Source: CAD feature listing. Evaluate the final solid. Frame: model axes, mm. A direction names the side the tool comes from. Round coordinates to 2 decimals unless told otherwise and drop trailing zeros. Loops run counter-clockwise (first coordinate to the right, second up) from the corner with the lowest first, then second, coordinate; pieces in that order, holes last. Notation, with made-up numbers: (-16, 48) -> (-1, 48) arc R28 ccw to (-1, 75) -> close; hole circle Ø9 at (81, -35.75). An arc over 180 degrees is marked (long way). Put each result on its own line as item: value. Start each with the question number.
1. Cut plane D-D (y = 7.5). Return the cut outline in (x, z), then the cut area to 3 significant figures.
2. Cut plane C-C (z = -1). State how many separate pieces and enclosed holes the cut face has, then the cut area to 3 significant figures.
3. Contact query for flat-ended pins moving along their axis: pin 1 (4 mm diameter, centred on y = -13.5, z = -3, fed in from +X); pin 2 (2.5 mm diameter, centred on x = -25, z = -3.5, fed in from -Y); pin 3 (4 mm diameter, centred on x = -26, z = -3, fed in from +Y). Output: stop coordinate, or through.
4. Cut plane B-B (x = -9). Return the cut outline in (y, z).
5. Draft query along Y for faces 1 (the cylindrical face through (21.37, 11.23, 8.55)), 2 (the cylindrical face through (-24.503, -13.631, 8.549)), 3 (the flat face through (0, -20, 4)), 4 (the cylindrical face through (-12.41, -16.07, 7.75)). Return one class per face: pulls with the +Y half, pulls with the -Y half, needs draft (parallel to the pull), parting line crosses it, or undercut.
6. Set-up query: faces 5 (the flat face through (10, 14, 3)), 6 (the flat face through (12.3, 4, 6.6)), 7 (the cylindrical face through (-7.9, -17.97, -1.09)). Return all of +Z, -Z, +X, -X, +Y, -Y with unobstructed straight access to the full face (end or side cutting, diameter ignored); none if empty.
7. Material intervals for L1, parallel to X at y = 13, z = -2; L2, parallel to X at y = -13, z = 0.5; L3, parallel to Y at x = -22.5, z = 8, sorted ascending.
8. Cut plane A-A (y = -1). Return the cut outline in (x, z), then the cut area to 3 significant figures.
```python
from build123d import *
from build123d.topology import SkipClean

# Parameters (mm, degrees)
ESQUISSE1_W                  = 55
ESQUISSE1_H                  = 45
BOSS_EXTRU_1_DEPTH           = 12
ESQUISSE2_R                  = 4.25
ENL_V_MAT_EXTRU_1_DEPTH      = 55.085580333
ENL_V_MAT_EXTRU_2_DEPTH      = 12.25
ENL_V_MAT_EXTRU_2_DEPTH_BACK = 12.25
ESQUISSE3_R                  = 7.75
ESQUISSE9_W                  = 61.062756781
ESQUISSE9_H                  = 12.22812859
ESQUISSE9_W_2                = 59.427147224
ESQUISSE9_H_2                = 8.100161614
ENL_V_MAT_EXTRU_7_DEPTH      = 31
SKETCH1_W                    = 55
SKETCH1_H                    = 36
BOSS_EXTRUDE1_DEPTH          = 5
SKETCH2_R                    = 2.1
CUT_EXTRUDE1_DEPTH           = 38.003378224
SKETCH3_R                    = 4
CUT_EXTRUDE2_DEPTH           = 10
CUT_EXTRUDE3_DEPTH           = 5
SKETCH5_R                    = 2.1
CUT_EXTRUDE4_DEPTH           = 47.864165415
BOSS_EXTRUDE4_START          = 2
SKETCH7_R                    = 2.1
BOSS_EXTRUDE4_DEPTH          = 2
SKETCH8_R                    = 2.1
BOSS_EXTRUDE5_DEPTH          = 2
SKETCH9_W                    = 7
SKETCH9_H                    = 3.2
CUT_EXTRUDE6_DEPTH           = 8
SKETCH10_W                   = 4.25
SKETCH10_H                   = 4
SKETCH10_H_2                 = 2
SKETCH10_H_3                 = 10
SKETCH10_W_2                 = 0.75


with BuildPart() as part:
    # Esquisse1 → Boss.-Extru.1 (new body)
    with BuildSketch(Plane.XY):
        Rectangle(ESQUISSE1_W, ESQUISSE1_H)
    extrude(amount=BOSS_EXTRU_1_DEPTH)

    # Esquisse2 → Enl_v. mat.-Extru.1 (cut, through all)
    with BuildSketch(Plane(origin=(0, 22.5, 0), x_dir=(1, 0, 0), z_dir=(0, 1, 0))):
        with Locations((-12.5, -12)):
            Circle(ESQUISSE2_R)
        with Locations((12.5, -12)):
            Circle(ESQUISSE2_R)
    extrude(amount=-ENL_V_MAT_EXTRU_1_DEPTH, mode=Mode.SUBTRACT)

    # Esquisse3 → Enl_v. mat.-Extru.2 (cut, two sides: drawn at the far end of the back side and taken through both)
    with BuildSketch(Plane(origin=(0, 0, 0), x_dir=(1, 0, 0), z_dir=(0, 1, 0)).offset(-ENL_V_MAT_EXTRU_2_DEPTH_BACK)):
        with Locations((-12.5, -12)):
            Circle(ESQUISSE3_R)
    extrude(amount=ENL_V_MAT_EXTRU_2_DEPTH + ENL_V_MAT_EXTRU_2_DEPTH_BACK, mode=Mode.SUBTRACT)

    # Esquisse9 → Enl_v. mat.-Extru.7 (cut)
    with BuildSketch(Plane.XY.offset(12)):
        with Locations((-0.389430846, -24.114064295)):
            Rectangle(ESQUISSE9_W, ESQUISSE9_H)
        with Locations((1.674552641, 22.050080807)):
            Rectangle(ESQUISSE9_W_2, ESQUISSE9_H_2)
    extrude(amount=-ENL_V_MAT_EXTRU_7_DEPTH, mode=Mode.SUBTRACT)

    # Sketch1 → Boss-Extrude1 (add)
    with BuildSketch(Plane(origin=(0, 0, 0), x_dir=(-1, 0, 0), z_dir=(0, 0, -1))):
        Rectangle(SKETCH1_W, SKETCH1_H)
    extrude(amount=BOSS_EXTRUDE1_DEPTH)

    # Sketch2 → Cut-Extrude1 (cut, through all)
    with BuildSketch(Plane.XY.offset(12)):
        with Locations((-22.5, 13)):
            Circle(SKETCH2_R)
        with Locations(Location((22.5, 13, 0), (0, 0, 180))):
            Circle(SKETCH2_R)
        with Locations((22.5, -13)):
            Circle(SKETCH2_R)
        with Locations(Location((-22.5, -13, 0), (0, 0, 180))):
            Circle(SKETCH2_R)
    extrude(amount=-CUT_EXTRUDE1_DEPTH, mode=Mode.SUBTRACT)

    # Sketch3 → Cut-Extrude2 (cut)
    with BuildSketch(Plane(origin=(0, 0, -5), x_dir=(-1, 0, 0), z_dir=(0, 0, -1))):
        with Locations((-22.5, 13)):
            Circle(SKETCH3_R)
        with Locations((22.5, 13)):
            Circle(SKETCH3_R)
        with Locations((22.5, -13)):
            Circle(SKETCH3_R)
        with Locations((-22.5, -13)):
            Circle(SKETCH3_R)
    extrude(amount=-CUT_EXTRUDE2_DEPTH, mode=Mode.SUBTRACT)

    # Sketch4 → Cut-Extrude3 (cut)
    with BuildSketch(Plane(origin=(0, 0, -5), x_dir=(-1, 0, 0), z_dir=(0, 0, -1))):
        with BuildLine():
            Line((-18.5, 13), (-18.5, 18))
            Line((-18.5, 18), (-27.5, 18))
            Line((-27.5, 18), (-27.5, 9))
            Line((-27.5, 9), (-22.5, 9))
            ThreePointArc((-22.5, 9), (-25.328427125, 15.828427125), (-18.5, 13))
        make_face()
        with BuildLine():
            Line((-22.5, -9), (-27.5, -9))
            Line((-27.5, -9), (-27.5, -18))
            Line((-27.5, -18), (-18.5, -18))
            Line((-18.5, -18), (-18.5, -13))
            ThreePointArc((-18.5, -13), (-25.328427125, -15.828427125), (-22.5, -9))
        make_face()
        with BuildLine():
            Line((27.5, -18), (27.5, -9))
            Line((27.5, -9), (22.5, -9))
            ThreePointArc((22.5, -9), (25.328427125, -15.828427125), (18.5, -13))
            Line((18.5, -13), (18.5, -18))
            Line((18.5, -18), (27.5, -18))
        make_face()
        with BuildLine():
            Line((27.5, 18), (18.5, 18))
            Line((18.5, 18), (18.5, 13))
            ThreePointArc((18.5, 13), (25.328427125, 15.828427125), (22.5, 9))
            Line((22.5, 9), (27.5, 9))
            Line((27.5, 9), (27.5, 18))
        make_face()
    extrude(amount=-CUT_EXTRUDE3_DEPTH, mode=Mode.SUBTRACT)

    # Sketch5 → Cut-Extrude4 (cut, through all)
    with BuildSketch(Plane(origin=(0, 18, 0), x_dir=(1, 0, 0), z_dir=(0, 1, 0))):
        with Locations(Location((-10, 1, 0), (0, 0, 180))):
            Circle(SKETCH5_R)
        with Locations(Location((10, 1, 0), (0, 0, 180))):
            Circle(SKETCH5_R)
    extrude(amount=-CUT_EXTRUDE4_DEPTH, mode=Mode.SUBTRACT)

    # Sketch7 → Boss-Extrude4 (add)
    with SkipClean():  # the faces are left unmerged after this step: merging them gives an invalid solid
        with BuildSketch(Plane(origin=(0, 18, 0), x_dir=(1, 0, 0), z_dir=(0, 1, 0)).offset(BOSS_EXTRUDE4_START)):
            with BuildLine():
                Line((18.5, 5), (-18.5, 5))
                Line((-18.5, 5), (-18.5, 0))
                Line((-18.5, 0), (-27.5, 0))
                Line((-27.5, 0), (-27.5, -12))
                Line((-27.5, -12), (-16.75, -12))
                ThreePointArc((-16.75, -12), (-12.5, -7.75), (-8.25, -12))
                Line((-8.25, -12), (8.25, -12))
                ThreePointArc((8.25, -12), (12.5, -7.75), (16.75, -12))
                Line((16.75, -12), (27.5, -12))
                Line((27.5, -12), (27.5, 0))
                Line((27.5, 0), (18.5, 0))
                Line((18.5, 0), (18.5, 5))
            make_face()
            with Locations(Location((10, 1, 0), (0, 0, 180))):
                Circle(SKETCH7_R, mode=Mode.SUBTRACT)
            with Locations(Location((-10, 1, 0), (0, 0, 180))):
                Circle(SKETCH7_R, mode=Mode.SUBTRACT)
        extrude(amount=-BOSS_EXTRUDE4_DEPTH)
    add(part.part.scale(1), mode=Mode.REPLACE)  # the faces are merged on a copy

    # Sketch8 → Boss-Extrude5 (add)
    with BuildSketch(Plane.XZ.offset(18)):
        with BuildLine():
            Line((-27.5, 0), (-18.5, 0))
            Line((-18.5, 0), (-18.5, -5))
            Line((-18.5, -5), (18.5, -5))
            Line((18.5, -5), (18.5, 0))
            Line((18.5, 0), (27.5, 0))
            Line((27.5, 0), (27.5, 12))
            Line((27.5, 12), (16.75, 12))
            ThreePointArc((16.75, 12), (12.5, 7.75), (8.25, 12))
            Line((8.25, 12), (-8.25, 12))
            ThreePointArc((-8.25, 12), (-12.5, 7.75), (-16.75, 12))
            Line((-16.75, 12), (-27.5, 12))
            Line((-27.5, 12), (-27.5, 0))
        make_face()
        with Locations(Location((10, -1, 0), (0, 0, 180))):
            Circle(SKETCH8_R, mode=Mode.SUBTRACT)
        with Locations(Location((-10, -1, 0), (0, 0, 180))):
            Circle(SKETCH8_R, mode=Mode.SUBTRACT)
    extrude(amount=BOSS_EXTRUDE5_DEPTH)

    # Sketch9 → Cut-Extrude6 (cut)
    with BuildSketch(Plane(origin=(0, 0, -5), x_dir=(-1, 0, 0), z_dir=(0, 0, -1))):
        with Locations((-10, 14.4)):
            Rectangle(SKETCH9_W, SKETCH9_H)
        with Locations((10, 14.4)):
            Rectangle(SKETCH9_W, SKETCH9_H)
        with Locations((10, -14.4)):
            Rectangle(SKETCH9_W, SKETCH9_H)
        with Locations((-10, -14.4)):
            Rectangle(SKETCH9_W, SKETCH9_H)
    extrude(amount=-CUT_EXTRUDE6_DEPTH, mode=Mode.SUBTRACT)

    # Sketch10 → Cut-Revolve1 (revolve, cut)
    with BuildSketch(Plane.XY.offset(12)):
        with Locations((14.625, 2)):
            Rectangle(SKETCH10_W, SKETCH10_H)
        with Locations((14.625, 5)):
            Rectangle(SKETCH10_W, SKETCH10_H_2)
        Polygon((16.75, 4), (16.75, 0), (17.5, 0), (23.5, 0), (23.5, 4), (17.5, 4), align=None)
        with Locations((14.625, -5)):
            Rectangle(SKETCH10_W, SKETCH10_H_3)
        with Locations((17.125, -5)):
            Rectangle(SKETCH10_W_2, SKETCH10_H_3)
        with Locations((17.125, 5)):
            Rectangle(SKETCH10_W_2, SKETCH10_H_2)
    revolve(axis=Axis((12.5, 20, 12), (0, -1, 0)), mode=Mode.SUBTRACT)


solid = part.part
```
Solution:
1. outline: (-27.5, -5) -> (27.5, -5) -> (27.5, 12) -> (16.75, 12) arc R4.25 cw to (8.25, 12) -> (-4.75, 12) arc R7.75 cw to (-20.25, 12) -> (-27.5, 12) -> close; hole circle Ø4.2 at (-10, -1); hole circle Ø4.2 at (10, -1)
1. area: 785 mm^2
2. separate pieces: 3
2. enclosed holes: 0
2. area: 1,450 mm^2
3. pin 1: stops at x = 18.79
3. pin 2: stops at y = -9
3. pin 3: stops at y = 9
4. outline: (-20, -5) -> (-16, -5) -> (-16, -2.85) -> (-20, -2.85) -> close; (-20, 0.85) -> (-16, 0.85) -> (-16, 3) -> (-12.8, 3) -> (-12.8, 0.85) -> (12.8, 0.85) -> (12.8, 3) -> (16, 3) -> (16, 0.85) -> (20, 0.85) -> (20, 9.59) -> (12.25, 9.59) -> (12.25, 5.09) -> (-12.25, 5.09) -> (-12.25, 9.59) -> (-20, 9.59) -> close; (-12.8, -5) -> (12.8, -5) -> (12.8, -2.85) -> (-12.8, -2.85) -> close; (16, -5) -> (20, -5) -> (20, -2.85) -> (16, -2.85) -> close
5. face 1: undercut
5. face 2: undercut
5. face 3: pulls with the -Y half
5. face 4: needs draft
6. face 5: -Z
6. face 6: +Z
6. face 7: +Y, -Y
7. L1: x = -18.5 to -13.5, -6.5 to 6.5, 13.5 to 18.5
7. L2: x = -27.5 to -26.5, -18.5 to -13.5, -6.5 to 6.5, 13.5 to 18.5, 26.5 to 27.5
7. L3: y = -20 to -15.1, -10.9 to 10.9, 15.1 to 20
8. outline: (-27.5, -5) -> (27.5, -5) -> (27.5, 12) -> (17.5, 12) arc R5 cw to (7.5, 12) -> (-4.75, 12) arc R7.75 cw to (-20.25, 12) -> (-27.5, 12) -> close; hole circle Ø4.2 at (-10, -1); hole circle Ø4.2 at (10, -1)
8. area: 774 mm^2
